from build123d import *

# Parameters (mm, degrees)
SZKIC1_W                    = 14.1
SZKIC1_H                    = 136.58
DODANIE_WYCI_GNI_CIE1_DEPTH = 6
PRZENIE_CIAN_1_BY           = 6
SZKIC3_W                    = 6.75
SZKIC3_H                    = 10.4
SZKIC3_W_2                  = 6.95
SZKIC3_H_2                  = 6.4
SZKIC3_H_3                  = 6.342942851
WYTNIJ_WYCI_GNI_CIE1_DEPTH  = 107.058352026
SZKIC4_R                    = 1.55
WYTNIJ_WYCI_GNI_CIE2_DEPTH  = 107.058352026
WYTNIJ_WYCI_GNI_CIE3_DEPTH  = 10


with BuildPart() as part:
    # Szkic1 → Dodanie-wyciągnięcie1 (new body)
    with BuildSketch(Plane.XY):
        with Locations((-72.400450183, 1.710000001)):
            Rectangle(SZKIC1_W, SZKIC1_H)
    extrude(amount=-DODANIE_WYCI_GNI_CIE1_DEPTH)

    # Przenieś ścianę1: a face moved inward by 6.0
    extrude(part.faces().sort_by_distance((-72.400450183, -66.579999999, -3))[0], amount=PRZENIE_CIAN_1_BY, dir=(0, 1, 0), mode=Mode.SUBTRACT)

    # Szkic3 → Wytnij-wyciągnięcie1 (cut, through all)
    with BuildSketch(Plane.XY):
        with Locations((-76.075450183, -37.590311709)):
            Rectangle(SZKIC3_W, SZKIC3_H)
        with Locations((-68.613894602, 67.000000001)):
            Rectangle(SZKIC3_W_2, SZKIC3_H_2)
        with Locations((-68.613894602, 27.000000001)):
            Rectangle(SZKIC3_W_2, SZKIC3_H_2)
        with Locations((-68.625450183, -57.608528574)):
            Rectangle(SZKIC3_W_2, SZKIC3_H_3)
        with Locations((-68.613894602, -17.579999999)):
            Rectangle(SZKIC3_W_2, SZKIC3_H_2)
        with Locations((-76.075450183, 47.000000001)):
            Rectangle(SZKIC3_W, SZKIC3_H)
    extrude(amount=-WYTNIJ_WYCI_GNI_CIE1_DEPTH, mode=Mode.SUBTRACT)

    # Szkic4 → Wytnij-wyciągnięcie2 (cut, through all)
    with BuildSketch(Plane.XY):
        with Locations((-75.450450183, 61.000000001)):
            Circle(SZKIC4_R)
        with Locations((-75.450450183, -51.579999999)):
            Circle(SZKIC4_R)
        with Locations((-75.450450183, 33.000000001)):
            Circle(SZKIC4_R)
        with Locations((-75.450450183, -23.579999999)):
            Circle(SZKIC4_R)
    extrude(amount=-WYTNIJ_WYCI_GNI_CIE2_DEPTH, mode=Mode.SUBTRACT)

    # Szkic5 → Wytnij-wyciągnięcie3 (cut)
    with BuildSketch(Plane(origin=(0, 0, -6), x_dir=(-1, 0, 0), z_dir=(0, 0, -1))):
        with BuildLine():
            Line((65.350450183, -0.745155849), (65.350450183, -8.845155849))
            Line((65.350450183, -8.845155849), (70.650450183, -8.845155849))
            ThreePointArc((70.650450183, -8.845155849), (74.700450183, -4.795155849), (70.650450183, -0.745155849))
            Line((70.650450183, -0.745155849), (65.350450183, -0.745155849))
        make_face()
        with BuildLine():
            Line((65.350450183, 10.154844151), (70.650450183, 10.154844151))
            ThreePointArc((70.650450183, 10.154844151), (74.700450183, 14.204844151), (70.650450183, 18.254844151))
            Line((70.650450183, 18.254844151), (65.350450183, 18.254844151))
            Line((65.350450183, 18.254844151), (65.350450183, 10.154844151))
        make_face()
    extrude(amount=-WYTNIJ_WYCI_GNI_CIE3_DEPTH, mode=Mode.SUBTRACT)


solid = part.part
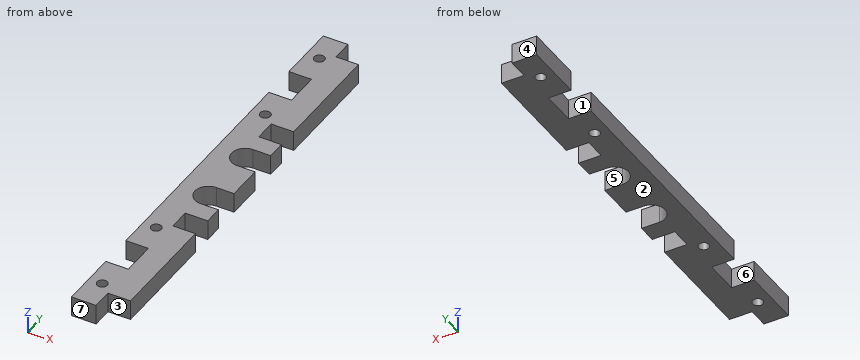
Geometry check sheet. Reference: the model listing, model coordinates, mm. Face numbers are marked on the shaded views. A direction names the side the tool comes from. Round coordinates to 2 decimals unless told otherwise and drop trailing zeros. Write each loop counter-clockwise with the first axis right and the second up, starting at its lowest first coordinate (ties: lowest second). Pieces come first, ordered by that corner, then holes. Notation, with made-up numbers: (61.5, -17) -> (107.5, -17) arc R27 ccw to (107.5, 14) -> close; hole circle Ø11 at (70.25, 86). An arc over 180 degrees is marked (long way). One line per item, written item: value. Start each with the question number.
(1) Cross-section at A-A, the plane y = 61. Record the cut outline in (x, z).
(2) Draft check along Y on the marked faces 1, 2, 3 and 4. Enter one of: +Y half, -Y half, draft (parallel to the pull), parting line (faces both ways), or undercut.
(3) Go/stop test with flat-tipped pins: pin 1 Ø1.6 at (x, z) = (-67, -2) entering from +Y; pin 2 Ø2.5 at (x, z) = (-68.5, -4.5) entering from -Y; pin 3 Ø3 at (y, z) = (66, -2.5) entering from +X. Record where each tip stops, or that it passes through.
(4) Cross-section at C-C, the plane z = -0.95. Give the number of separate pieces and of enclosed holes in the cut face, and give its area (3 significant figures).
(5) Scan lines: line 1 (Y direction, x = -77.25, z = -3.5); line 2 (Y direction, x = -68.75, z = -0.95); line 3 (Y direction, x = -73.75, z = -0.5). Record each from-to range of solid material in increasing order. Write a range as [from, to].
(6) Cross-section at B-B, the plane x = -67.5. Record the cut outline in (y, z), and give its area (3 significant figures).
(7) Access from +Z, -Z, +X, -X, +Y, -Y to the whole of each face (thin tool, end or side, straight path). Record for the marked faces 5, 6 and 7.
Answer:
1. outline: (-79.45, -6) -> (-77, -6) -> (-77, 0) -> (-79.45, 0) -> close; (-73.9, -6) -> (-65.35, -6) -> (-65.35, 0) -> (-73.9, 0) -> close
2. face 1: undercut
2. face 2: draft
2. face 3: -Y half
2. face 4: +Y half
3. pin 1: y = 63.8
3. pin 2: y = -54.44
3. pin 3: x = -72.09
4. separate pieces: 1
4. enclosed holes: 4
4. area: 1,360 mm²
5. line 1: [-60.58, -42.79], [-32.39, 41.8], [52.2, 70]
5. line 2: [-54.44, -20.78], [-14.38, -8.85], [-0.75, 10.15], [18.25, 23.8], [30.2, 63.8]
5. line 3: [-60.58, -42.79], [-32.39, -7.4], [-2.19, 11.6], [16.81, 41.8], [52.2, 70]
6. outline: (-54.44, -6) -> (-20.78, -6) -> (-20.78, 0) -> (-54.44, 0) -> close; (-14.38, -6) -> (-8.85, -6) -> (-8.85, 0) -> (-14.38, 0) -> close; (-0.75, -6) -> (10.15, -6) -> (10.15, 0) -> (-0.75, 0) -> close; (18.25, -6) -> (23.8, -6) -> (23.8, 0) -> (18.25, 0) -> close; (30.2, -6) -> (63.8, -6) -> (63.8, 0) -> (30.2, 0) -> close
6. area: 535 mm²
7. face 5: +Z, -Z, +X
7. face 6: +Z, -Z, -X
7. face 7: +Z, -Z, +X, -X, -Y
